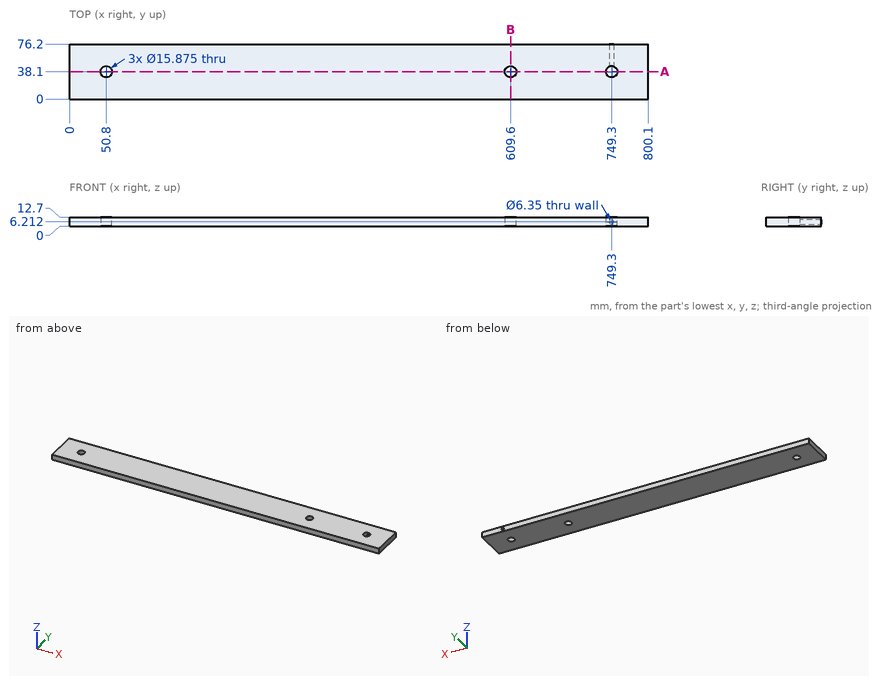
Geometry: see drawing. Coordinates: mm, zero at the bounding-box minimum. Round coordinates to 2 decimals unless told otherwise and drop trailing zeros. Loops run counter-clockwise (first coordinate to the right, second up) from the corner with the lowest first, then second, coordinate; pieces in that order, holes last. Notation, with made-up numbers: (14.5, 20) -> (41.5, 20) arc R33 ccw to (41.5, 54) -> close; hole circle Ø9 at (73, -22.75). An arc over 180 degrees is marked (long way). Use one line per item in the form item = value. Start each with the question number.
Item 1: Section query B-B on x = 609.6. Return the cut outline in (y, z).
Item 2: Section query A-A on y = 38.1. Return the cut outline in (x, z).
Item 3: Material intervals for L1, parallel to X at y = 38.1, z = 10.25; L2, parallel to X at y = 56, z = 6.5; L3, parallel to Y at x = 50.8, z = 5.5, sorted ascending. Write a range as from..to.
Item 4: Contact query for a flat-ended pin moving along its axis: pin 1 Ø18.5 at (x, y) = (609.6, 38.1) entering from -Z. Output: stop coordinate, or through.
Ans:
q1.outline = (0, 0) -> (30.16, 0) -> (30.16, 12.7) -> (0, 12.7) -> close; (46.04, 0) -> (76.2, 0) -> (76.2, 12.7) -> (46.04, 12.7) -> close
q2.outline = (0, 0) -> (42.86, 0) -> (42.86, 12.7) -> (0, 12.7) -> close; (58.74, 0) -> (601.66, 0) -> (601.66, 12.7) -> (58.74, 12.7) -> close; (617.54, 0) -> (741.36, 0) -> (741.36, 12.7) -> (617.54, 12.7) -> close; (757.24, 0) -> (800.1, 0) -> (800.1, 12.7) -> (757.24, 12.7) -> close
q3.L1 = 0..42.86, 58.74..601.66, 617.54..741.36, 757.24..800.1
q3.L2 = 0..746.14, 752.46..800.1
q3.L3 = 0..30.16, 46.04..76.2
q4.pin_1 = 0
